Design review of the part built by this model. Coordinates are the model's own, in mm. Round coordinates to 2 decimals unless told otherwise and drop trailing zeros. Order: outer loops, then holes, each group sorted by start corner. A loop starts at its lowest first (then second) coordinate and runs counter-clockwise, first axis right, second up. Notation, with made-up numbers: (87.25, -13.75) - (138.25, -13.75) arc R13 ccw to (138.25, 3.25) - close; hole circle Ø11 at (-36, 35.5). An arc over 180 degrees is marked (long way). Write item = value, one per line.
from build123d import *

# Parameters (mm, degrees)
SKETCH_1_W          = 95
SKETCH_1_H          = 150
EXTRUDE_1_DEPTH     = 4
SKETCH_2_R          = 3
CUT_EXTRUDE_1_DEPTH = 89.866472868


with BuildPart() as part:
    # 草图1 → 凸台-拉伸1 (new body)
    with BuildSketch(Plane.XY):
        Rectangle(SKETCH_1_W, SKETCH_1_H)
    extrude(amount=EXTRUDE_1_DEPTH)

    # 草图2 → 切除-拉伸1 (cut, through all)
    with BuildSketch(Plane.XY.offset(4)):
        with Locations((-39.5, 64)):
            Circle(SKETCH_2_R)
        with Locations((-15.5, 64)):
            Circle(SKETCH_2_R)
    cut_extrude_1 = extrude(amount=-CUT_EXTRUDE_1_DEPTH, mode=Mode.SUBTRACT)

    # 镜向1: 切除-拉伸1 across plane
    add(cut_extrude_1.mirror(Plane(origin=(0, 0, 0), x_dir=(0, 0, 1), z_dir=(1, 0, 0))), mode=Mode.SUBTRACT)


solid = part.part
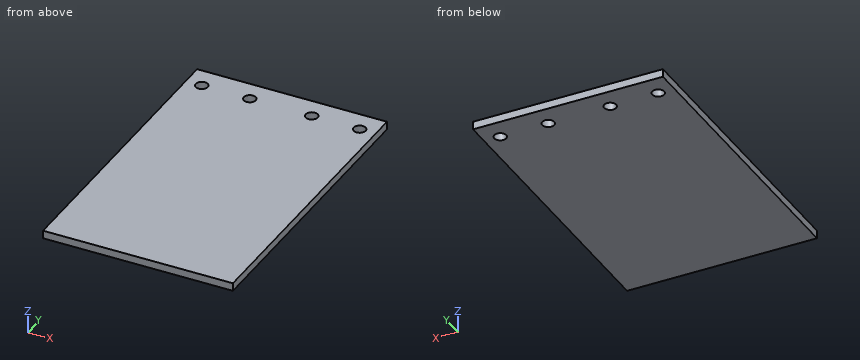
Item 1: Take a section at A-A, the plane x = 15.5. State the section outline as (y, z) points, and give its area (3 significant figures).
Data:
outline = (-75, 0) - (61, 0) - (61, 4) - (-75, 4) - close; (67, 0) - (75, 0) - (75, 4) - (67, 4) - close
area = 576 mm2
Item 2: Take a section at B-B, the plane y = 64. State the section outline as (x, z) points.
Data:
outline = (-47.5, 0) - (-42.5, 0) - (-42.5, 4) - (-47.5, 4) - close; (-36.5, 0) - (-18.5, 0) - (-18.5, 4) - (-36.5, 4) - close; (-12.5, 0) - (12.5, 0) - (12.5, 4) - (-12.5, 4) - close; (18.5, 0) - (36.5, 0) - (36.5, 4) - (18.5, 4) - close; (42.5, 0) - (47.5, 0) - (47.5, 4) - (42.5, 4) - close
Item 3: For line 1 along Y through (x, z) = (39.5, 2); line 2 along Y through (x, z) = (-41, 1.05), list the stretches that pass through material, from the lowest coordinate up. Write a range as [from, to].
Data:
line_1 = [-75, 61], [67, 75]
line_2 = [-75, 61.4], [66.6, 75]
Item 4: Insertion check: P1, Ø3.5, axis at x = 39.5, y = 64, coming from the -Z side; P2, Ø8, axis at x = -15.5, y = 64, coming from the +Z side. Each pin has a flat end and moves straight along its axis. Give the tip position at first contact, or say it passes through.
Data:
P1 = through
P2 = 4
